Could you check a few things on this drawing? It's one solid part, dimensions in mm from its lowest x, y, z. A direction names the side the tool comes from. Give positions to 0.01 mm unless a question says otherwise; leave off trailing zeros. Loops run counter-clockwise (first coordinate to the right, second up) from the corner with the lowest first, then second, coordinate; pieces in that order, holes last. Notation, with made-up numbers: M 58.5,70 L 111.5,70 A14 ccw 111.5,94 Z; hole C 26,-39 d2. An arc over 180 degrees is marked long. Answer in a Markdown table with one row per item. Add a question column.
1. I need wall thicknesses on line 1 along Y through (x, z) = (81, 23) (1 decimal); line 2 along Y through (x, z) = (14.5, 43); line 3 along Y through (x, z) = (105, 4.5) (1 decimal). Which ranges of each line are inside material? Lowest first, please. Write a range as from..to.
2. If we section it at B-B on y = 5: List the corners of the cut face in (x, z) for me (1 decimal).
3. If we section it at D-D on z = 8.5: List the corners of the cut face in (x, y) for me (1 decimal).
4. If we section it at C-C on x = 97.5: List the corners of the cut face in (y, z) for me (1 decimal).
5. Thinking about a two-plate mould opening in X: for the marked faces 4, 5, 6 and 7, which applies, released by +X, released by -X, zero draft, split by the parting line, or undercut?
6. If we section it at A-A on y = 55: List the corners of the cut face in (x, z) for me (1 decimal).
7. Which directions (+Z, -Z, +X, -X, +Y, -Y) give clear straight access to the entire face, cutting with the end or side of a thin tool? Please do the marked faces 1, 2 and 3.
8. I'm going to push flat-ended pins straight in: pin 1 Ø10 at (x, z) = (89, 7) entering from -Y; pin 2 Ø3.5 at (y, z) = (21, 5) entering from -X; pin 3 Ø8.5 at (y, z) = (5.5, 23) entering from +X; pin 4 Ø6 at (x, y) = (80.52, 56.64) entering from -Z. Where does each tip first touch, or does it pass through?
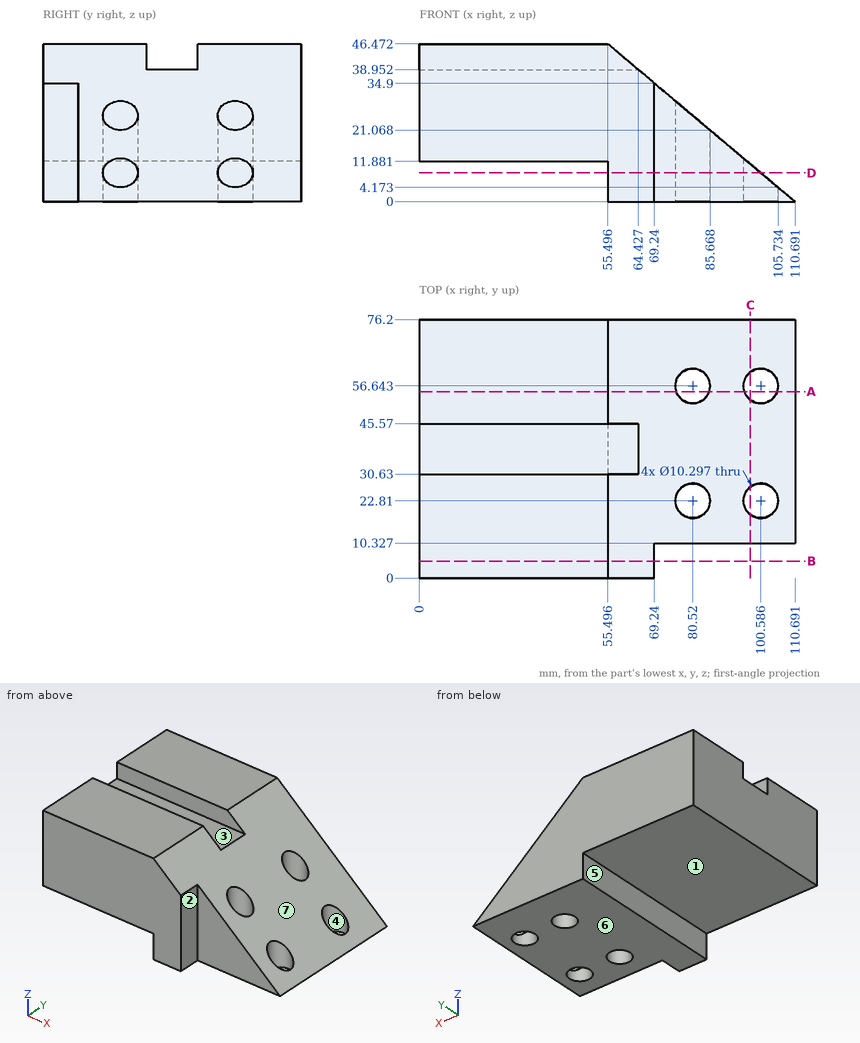
Results:
| question | item | result |
|---|---|---|
| 1 | line 1 | 10.3..17.7, 27.9..51.5, 61.8..76.2 |
| 1 | line 2 | 0..30.63, 45.57..76.2 |
| 1 | line 3 | 10.3..20.2, 25.5..54, 59.3..76.2 |
| 2 | outline | M 0,11.9 L 55.5,11.9 L 55.5,0 L 69.2,0 L 69.2,34.9 L 55.5,46.5 L 0,46.5 Z |
| 3 | outline | M 55.5,0 L 69.2,0 L 69.2,10.3 L 100.6,10.3 L 100.6,17.7 A5.1 cw 100.6,28 L 100.6,51.5 A5.1 cw 100.6,61.8 L 100.6,76.2 L 55.5,76.2 Z; hole C 80.5,22.8 d10.3; hole C 80.5,56.6 d10.3 |
| 4 | outline | M 10.3,0 L 18.7,0 L 18.7,11.1 L 10.3,11.1 Z; M 26.9,0 L 52.5,0 L 52.5,11.1 L 26.9,11.1 Z; M 60.8,0 L 76.2,0 L 76.2,11.1 L 60.8,11.1 Z |
| 5 | face 4 | undercut |
| 5 | face 5 | released by -X |
| 5 | face 6 | zero draft |
| 5 | face 7 | released by +X |
| 6 | outline | M 0,11.9 L 55.5,11.9 L 55.5,0 L 75.6,0 L 75.6,29.5 L 55.5,46.5 L 0,46.5 Z; M 85.4,0 L 95.7,0 L 95.7,12.6 L 85.4,21.3 Z; M 105.5,0 L 110.7,0 L 105.5,4.4 Z |
| 7 | face 1 | -Z, -X, +Y, -Y |
| 7 | face 2 | +Z, -Z, +X, -Y |
| 7 | face 3 | +Z, +X, -X |
| 8 | pin 1 | y = 10.33 |
| 8 | pin 2 | x = 55.5 |
| 8 | pin 3 | x = 69.24 |
| 8 | pin 4 | through |
